Check sheet for the drawn part. Datum: minimum x, y, z corner. Units: mm. A direction names the side the tool comes from. Coordinates: 2 decimals unless noted, no trailing zeros. Write each loop counter-clockwise with the first axis right and the second up, starting at its lowest first coordinate (ties: lowest second). Pieces come first, ordered by that corner, then holes. Notation, with made-up numbers: (45.5, 30.25) -> (57.5, 30.25) arc R17 cw to (57.5, 55.25) -> close; hole circle Ø8 at (14, 11). An arc over 180 degrees is marked (long way). Answer in a Markdown table with one row per item. Add a question column.
Q1. Section check A-A, the plane y = 12. Record the boundary of the cut face in (x, z).
Q2. Section check C-C, the plane x = 12. Record the boundary of the cut face in (y, z), and give its area (3 significant figures).
Q3. Release check for a two-part mould opening along Y. For the marked faces 1, 2, 3 and 4 record: pulls with the +Y half, pulls with the -Y half, needs draft (parallel to the pull), parting line crosses it, or undercut.
Q4. Tool access check on the marked faces 5, 6 and 7. Record the directions out of +Z, -Z, +X, -X, +Y, -Y that give a thin tool (end or side, any length) a straight path to the whole face; none if there is none.
Q5. Section check D-D, the plane x = 21.5. Record the boundary of the cut face in (y, z).
Q6. Section check B-B, the plane z = 3.25. Record the boundary of the cut face in (x, y).
Q7. Gauge pin test, flat ends, axial feed: P1, Ø5, axis at x = 9, z = 5.5, coming from the -Y side; P2, Ø4, axis at x = 5.5, y = 3.5, coming from the +Z side; P3, Ø4, axis at x = 19.5, z = 2, coming from the -Y side (1 decimal). Record the tip position at first contact, or that the pin passes through.
Q8. Thickness scan on line 1 (Y direction, x = 12, z = 3.75); line 2 (X direction, y = 6, z = 3.75); line 3 (Y direction, x = 3.75, z = 6.5) (1 decimal). Record the ranges inside material, lowest first.
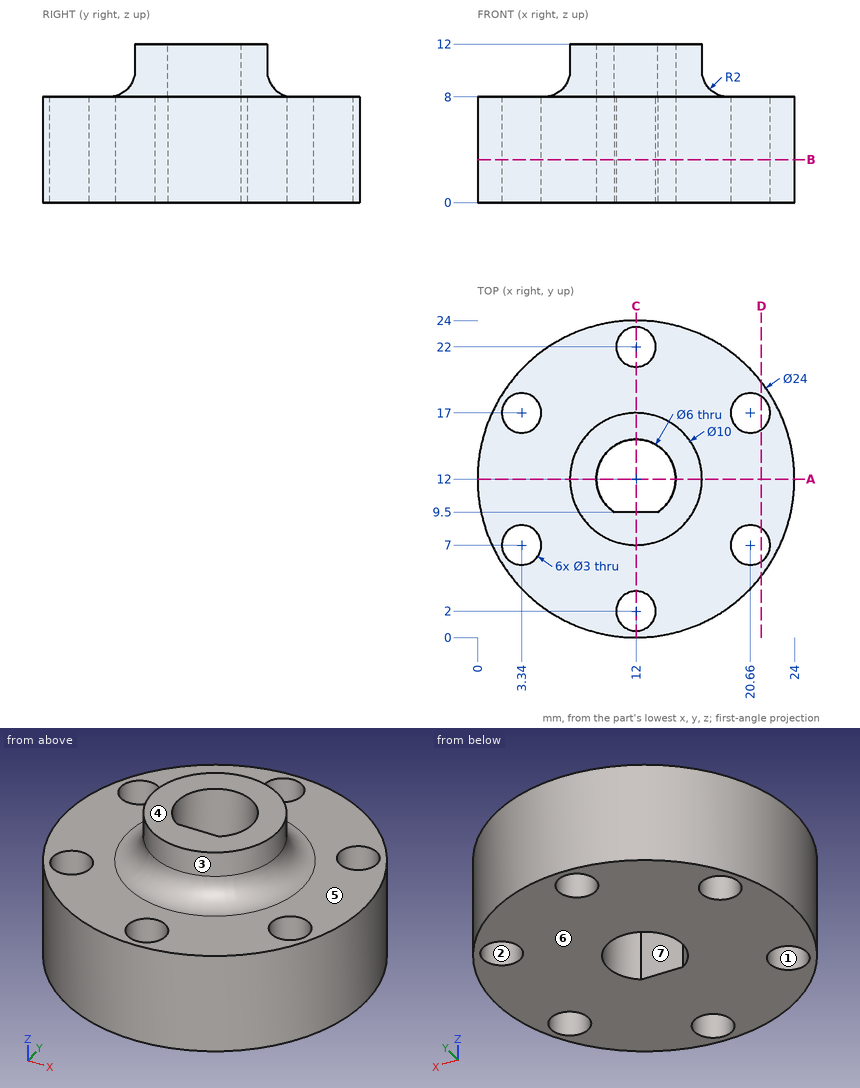
Calculated:
| question | item | result |
|---|---|---|
| 1 | outline | (0, 0) -> (9, 0) -> (9, 12) -> (7, 12) -> (7, 10) arc R2 cw to (5, 8) -> (0, 8) -> close; (15, 0) -> (24, 0) -> (24, 8) -> (19, 8) arc R2 cw to (17, 10) -> (17, 12) -> (15, 12) -> close |
| 2 | outline | (0, 0) -> (0.5, 0) -> (0.5, 8) -> (0, 8) -> close; (3.5, 0) -> (9.5, 0) -> (9.5, 12) -> (7, 12) -> (7, 10) arc R2 cw to (5, 8) -> (3.5, 8) -> close; (15, 0) -> (20.5, 0) -> (20.5, 8) -> (19, 8) arc R2 cw to (17, 10) -> (17, 12) -> (15, 12) -> close; (23.5, 0) -> (24, 0) -> (24, 8) -> (23.5, 8) -> close |
| 2 | area | 120 mm² |
| 3 | face 1 | undercut |
| 3 | face 2 | undercut |
| 3 | face 3 | parting line crosses it |
| 3 | face 4 | needs draft |
| 4 | face 5 | +Z |
| 4 | face 6 | -Z, +X, -X, +Y, -Y |
| 4 | face 7 | +Z, -Z |
| 5 | outline | (4.67, 0) -> (5.76, 0) -> (5.76, 8) -> (4.67, 8) -> close; (8.24, 0) -> (15.76, 0) -> (15.76, 8) -> (8.24, 8) -> close; (18.24, 0) -> (19.33, 0) -> (19.33, 8) -> (18.24, 8) -> close |
| 6 | outline | circle Ø24 at (12, 12); hole circle Ø3 at (3.34, 7); hole circle Ø3 at (3.34, 17); hole (10.34, 9.5) -> (13.66, 9.5) arc R3 ccw (long way) to start; hole circle Ø3 at (12, 2); hole circle Ø3 at (12, 22); hole circle Ø3 at (20.66, 7); hole circle Ø3 at (20.66, 17) |
| 7 | P1 | stops at y = 0.01 |
| 7 | P2 | stops at z = 8 |
| 7 | P3 | stops at y = 1.3 |
| 8 | line 1 | y = 0 to 0.5, 3.5 to 9.5, 15 to 20.5, 23.5 to 24 |
| 8 | line 2 | x = 1.61 to 2.22, 4.46 to 19.54, 21.78 to 22.39 |
| 8 | line 3 | y = 3.3 to 5.6, 8.4 to 15.6, 18.4 to 20.7 |
